from build123d import *

# Parameters (mm, degrees)
SKETCH_1_R               = 85
SKETCH_1_R_2             = 10.5
EXTRUDE_1_DEPTH          = 6
SKETCH_2_R               = 2
CUT_EXTRUDE_1_DEPTH      = 3
PATTERN_CIRCULAR_2_COUNT = 4
CHAMFER_1_SIZE           = 3


with BuildPart() as part:
    # 草图1 → 凸台-拉伸1 (new body)
    with BuildSketch(Plane.XY):
        Circle(SKETCH_1_R)
        with BuildLine():
            Line((-31.725622255, -22.214519858), (-52.610992631, -36.838613633))
            ThreePointArc((-52.610992631, -36.838613633), (-60.837871991, -38.331841306), (-67.323181147, -33.054338296))
            ThreePointArc((-67.323181147, -33.054338296), (-75, 0), (-67.323181147, 33.054338296))
            ThreePointArc((-67.323181147, 33.054338296), (-60.837871991, 38.331841306), (-52.610992631, 36.838613633))
            Line((-52.610992631, 36.838613633), (-31.725622255, 22.214519858))
            ThreePointArc((-31.725622255, 22.214519858), (-27.910605416, 16.986540946), (-28.096039964, 10.517249561))
            ThreePointArc((-28.096039964, 10.517249561), (-30, 0), (-28.096039964, -10.517249561))
            ThreePointArc((-28.096039964, -10.517249561), (-27.910605416, -16.986540946), (-31.725622255, -22.214519858))
        make_face(mode=Mode.SUBTRACT)
        with BuildLine():
            Line((22.214519858, -31.725622255), (36.838613633, -52.610992631))
            ThreePointArc((36.838613633, -52.610992631), (38.331841306, -60.837871991), (33.054338296, -67.323181147))
            ThreePointArc((33.054338296, -67.323181147), (0, -75), (-33.054338296, -67.323181147))
            ThreePointArc((-33.054338296, -67.323181147), (-38.331841306, -60.837871991), (-36.838613633, -52.610992631))
            Line((-36.838613633, -52.610992631), (-22.214519858, -31.725622255))
            ThreePointArc((-22.214519858, -31.725622255), (-16.986540946, -27.910605416), (-10.517249561, -28.096039964))
            ThreePointArc((-10.517249561, -28.096039964), (0, -30), (10.517249561, -28.096039964))
            ThreePointArc((10.517249561, -28.096039964), (16.986540946, -27.910605416), (22.214519858, -31.725622255))
        make_face(mode=Mode.SUBTRACT)
        with BuildLine():
            Line((36.838613633, 52.610992631), (22.214519858, 31.725622255))
            ThreePointArc((22.214519858, 31.725622255), (16.986540946, 27.910605416), (10.517249561, 28.096039964))
            ThreePointArc((10.517249561, 28.096039964), (0, 30), (-10.517249561, 28.096039964))
            ThreePointArc((-10.517249561, 28.096039964), (-16.986540946, 27.910605416), (-22.214519858, 31.725622255))
            Line((-22.214519858, 31.725622255), (-36.838613633, 52.610992631))
            ThreePointArc((-36.838613633, 52.610992631), (-38.331841306, 60.837871991), (-33.054338296, 67.323181147))
            ThreePointArc((-33.054338296, 67.323181147), (0, 75), (33.054338296, 67.323181147))
            ThreePointArc((33.054338296, 67.323181147), (38.331841306, 60.837871991), (36.838613633, 52.610992631))
        make_face(mode=Mode.SUBTRACT)
        with BuildLine():
            Line((31.725622255, 22.214519858), (52.610992631, 36.838613633))
            ThreePointArc((52.610992631, 36.838613633), (60.837871991, 38.331841306), (67.323181147, 33.054338296))
            ThreePointArc((67.323181147, 33.054338296), (75, 0), (67.323181147, -33.054338296))
            ThreePointArc((67.323181147, -33.054338296), (60.837871991, -38.331841306), (52.610992631, -36.838613633))
            Line((52.610992631, -36.838613633), (31.725622255, -22.214519858))
            ThreePointArc((31.725622255, -22.214519858), (27.910605416, -16.986540946), (28.096039964, -10.517249561))
            ThreePointArc((28.096039964, -10.517249561), (30, 0), (28.096039964, 10.517249561))
            ThreePointArc((28.096039964, 10.517249561), (27.910605416, 16.986540946), (31.725622255, 22.214519858))
        make_face(mode=Mode.SUBTRACT)
        Circle(SKETCH_1_R_2, mode=Mode.SUBTRACT)
    extrude(amount=EXTRUDE_1_DEPTH)

    # 草图2 → 切除-拉伸1 (cut)
    with BuildSketch(Plane.XY.offset(6)):
        with Locations((0, 14.5)):
            Circle(SKETCH_2_R)
    cut_extrude_1 = extrude(amount=-CUT_EXTRUDE_1_DEPTH, mode=Mode.SUBTRACT)

    # 阵列(圆周)2: 切除-拉伸1 ×4 about axis
    pattern_circular_2_axis = Axis((0, 0, 0), (0, 0, 1))
    for i in range(1, PATTERN_CIRCULAR_2_COUNT):
        add(cut_extrude_1.rotate(pattern_circular_2_axis, i * 360 / PATTERN_CIRCULAR_2_COUNT), mode=Mode.SUBTRACT)

    # 倒角1
    chamfer_1_edges = [part.edges().sort_by_distance(p)[0] for p in [
        (-85, 0, 6),
    ]]
    chamfer(chamfer_1_edges, length=CHAMFER_1_SIZE)


solid = part.part
Build history of the part. All positions in model axes, mm. A direction names the side the tool comes from. Round coordinates to 2 decimals unless told otherwise and drop trailing zeros. Write each loop counter-clockwise with the first axis right and the second up, starting at its lowest first coordinate (ties: lowest second). Pieces come first, ordered by that corner, then holes. Notation, with made-up numbers: (79, 6) -> (97, 6) arc R25 ccw to (97, 42) -> close; hole circle Ø10 at (86.5, -15). An arc over 180 degrees is marked (long way). Use one line per item in the form item = value.
Q1. Two-plate mould, pull along Y, no slides. Class faces 1 (the cylindrical face through (27.884, 16.898, 2.958)), 2 (the conical face through (-17.808, -80.192, 5.854)), 3 (the flat face through (-20, 1, 0)): released by +Y, released by -Y, zero draft, split by the parting line, or undercut.
Conclusion:
face_1 = undercut
face_2 = split by the parting line
face_3 = zero draft
Q2. Drop flat-ended pins along their axis: P1, Ø4.5, axis at x = 0, y = 14.5, coming from the +Z side; P2, Ø1.2, axis at x = 15.5, y = 0.5, coming from the +Z side; P3, Ø1.5, axis at y = 29, z = 5.5, coming from the +X side; P4, Ø1.5, axis at y = -66, z = 3.5, coming from the +X side. Give the stop position or say it passes through.
Conclusion:
P1 = 6
P2 = 3
P3 = 78.08
P4 = 54.24
Q3. Drill centre lines: L1, parallel to Y at x = -25.5, z = 4; L2, parallel to X at y = -9.5, z = 3.45; L3, parallel to Y at x = 32.5, z = 2.5. Where is each one in solid material? Low to high.
Conclusion:
L1 = -80.04 to -70.53, -36.42 to 36.42, 70.53 to 80.04
L2 = -84.01 to -74.4, -28.46 to -4.47, 4.47 to 28.46, 74.4 to 84.01
L3 = -78.54 to -67.59, -46.41 to -22.76, 22.76 to 46.41, 67.59 to 78.54
Q4. Tool access for faces 4 (the cylindrical face through (-60.72, -38.36, 2.96)), 5 (the flat face through (-15, 0, 3)): list every direction of +Z, -Z, +X, -X, +Y, -Y with a clear straight run to the whole face (end or side of a thin tool).
Conclusion:
face_4 = +Z, -Z
face_5 = +Z
Q5. Band-saw the part on C-C, the plane z = 2.1. State how many separate pieces and enclosed holes the cut face has, then the cut area to 3 significant figures.
Conclusion:
separate_pieces = 1
enclosed_holes = 5
area = 11,100 mm²
Q6. Band-saw the part on A-A, the plane x = 0. Write the cut outline in (y, z), then the cut area to 3 significant figures.
Conclusion:
outline = (-85, 0) -> (-75, 0) -> (-75, 6) -> (-82, 6) -> (-85, 3) -> close; (-30, 0) -> (-10.5, 0) -> (-10.5, 6) -> (-12.5, 6) -> (-12.5, 3) -> (-16.5, 3) -> (-16.5, 6) -> (-30, 6) -> close; (10.5, 0) -> (30, 0) -> (30, 6) -> (16.5, 6) -> (16.5, 3) -> (12.5, 3) -> (12.5, 6) -> (10.5, 6) -> close; (75, 0) -> (85, 0) -> (85, 3) -> (82, 6) -> (75, 6) -> close
area = 321 mm²
